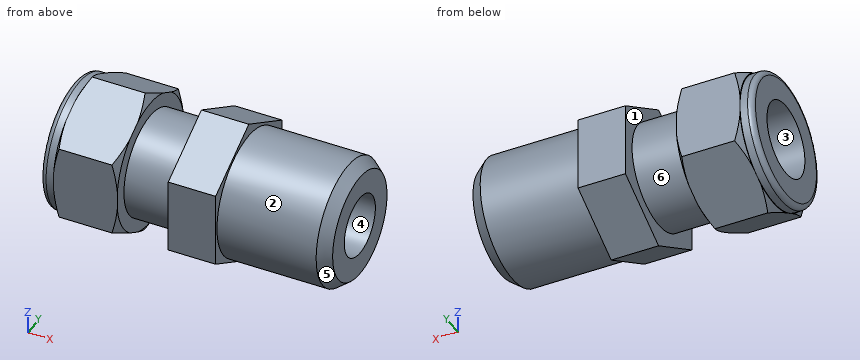
from build123d import *

# Parameters (mm, degrees)
HEX1_DEPTH         = 5.461
BODYFILLET_R       = 0.889
HEX2_DEPTH         = 8.128
DSCH_R             = 6.35
CUT_EXTRUDED_DEPTH = 22.86
SKETCH_E_R         = 5.207
CUT_EXTRUDEE_DEPTH = 26.162


with BuildPart() as part:
    # BodySch → Body (revolve)
    with BuildSketch(Plane.XY, mode=Mode.PRIVATE) as body_sk:
        Polygon((-49.022, 0), (-49.022, 11.1125), (-41.3766, 11.1125), (-41.3766, 8.89), (-27.178, 8.89), (-27.178, 10.668), (-2.033448841, 10.668), (0, 9.107679825), (0, 0), align=None)
    revolve(body_sk.sketch.rotate(Axis((-103.68469285, 0, 0), (1, 0, 0)), 90), axis=Axis((-103.68469285, 0, 0), (1, 0, 0)))

    # Hex1Sch_G → Hex1 (add, symmetric)
    with BuildSketch(Plane(origin=(-41.3766, 0, 0), x_dir=(0, 0, -1), z_dir=(1, 0, 0))):
        Polygon((12.831609733, 0), (6.415804866, 11.1125), (-6.415804866, 11.1125), (-12.831609733, 0), (-6.415804866, -11.1125), (6.415804866, -11.1125), align=None)
    extrude(amount=HEX1_DEPTH, both=True)

    # BodyFillet
    bodyfillet_edges = [part.edges().sort_by_distance(p)[0] for p in [
        (-49.022, 0, -11.1125),
    ]]
    fillet(bodyfillet_edges, radius=BODYFILLET_R)

    # HexfilletSch → Hexfillet (revolve, cut)
    with BuildSketch(Plane(origin=(0, 0, 0), x_dir=(1, 0, 0), z_dir=(0, 1, 0)), mode=Mode.PRIVATE) as hexfillet_sk:
        Polygon((-46.8376, 11.227658516), (-45.911558333, 12.831609733), (-46.8376, 12.831609733), align=None)
        Polygon((-35.9156, 11.227658516), (-36.841641667, 12.831609733), (-35.9156, 12.831609733), align=None)
    revolve(hexfillet_sk.sketch.rotate(Axis((-41.994761709, 0, 0), (1, 0, 0)), 150), axis=Axis((-41.994761709, 0, 0), (1, 0, 0)), mode=Mode.SUBTRACT)

    # Hex2Sch_F → Hex2 (add)
    with BuildSketch(Plane.ZY.offset(27.178)):
        Polygon((12.831609733, 0), (6.415804866, 11.1125), (-6.415804866, 11.1125), (-12.831609733, 0), (-6.415804866, -11.1125), (6.415804866, -11.1125), align=None)
    extrude(amount=-HEX2_DEPTH)

    # DSch → Cut-ExtrudeD (cut)
    with BuildSketch(Plane(origin=(-49.022, 0, 0), x_dir=(0, 0, -1), z_dir=(1, 0, 0))):
        Circle(DSCH_R)
    extrude(amount=CUT_EXTRUDED_DEPTH, mode=Mode.SUBTRACT)

    # Sketch E → Cut-ExtrudeE (cut)
    with BuildSketch(Plane(origin=(0, 0, 0), x_dir=(0, 0, -1), z_dir=(1, 0, 0))):
        Circle(SKETCH_E_R)
    extrude(amount=-CUT_EXTRUDEE_DEPTH, mode=Mode.SUBTRACT)


solid = part.part
Check sheet for the modelled part. Datum: model origin and axes. Units: mm. Face numbers are marked on the shaded views. A direction names the side the tool comes from. Round coordinates to 2 decimals unless told otherwise and drop trailing zeros. Write each loop counter-clockwise with the first axis right and the second up, starting at its lowest first coordinate (ties: lowest second). Pieces come first, ordered by that corner, then holes. Notation, with made-up numbers: (14.25, 83) - (21.25, 83) arc R14 ccw to (21.25, 106) - close; hole circle Ø10 at (23, 67). An arc over 180 degrees is marked (long way). Return JSON: item names as keys, results as strings.
Q1. Depth check by flat-ended pin: P1, Ø12, axis at x = -36, z = -4.5, coming from the -Y side; P2, Ø11.5, axis at y = 0, z = 0, coming from the -X side; P3, Ø12, axis at x = -42.5, y = 8.5, coming from the -Z side; P4, Ø1, axis at x = -27.5, y = 5, coming from the +Z side. Enter the tip coordinate at first touch or a pass-through.
Returned:
{"P1": "stops at y = -11.11", "P2": "stops at x = -26.16", "P3": "stops at z = -11.39", "P4": "stops at z = 10.17"}
Q2. Cross-section at B-B (x = -9). Record the boundary of the cut face in (y, z), then the cut area to 3 significant figures.
Returned:
{"outline": "circle Ø21.34 at (0, 0); hole circle Ø10.41 at (0, 0)", "area": "272 mm²"}
Q3. Scan lines: L1, parallel to Y at x = -10.5, z = -0.25; L2, parallel to Y at x = -20, z = 0; L3, parallel to X at y = -2.25, z = -4.75. Record each from-to range of solid material in increasing order. Write a range as from..to.
Returned:
{"L1": "y = -10.67..-5.2, 5.2..10.67", "L2": "y = -11.11..-5.21, 5.21..11.11", "L3": "x = -26.16..0"}
Q4. Access from +Z, -Z, +X, -X, +Y, -Y to the whole of each face (thin tool, end or side, straight path). Record for the marked faces 1, 2 and 3.
Returned:
{"face 1": "none", "face 2": "+X", "face 3": "-X"}
Q5. Draft check along X on the marked faces 4, 5 and 6. Enter one of: released by +X, released by -X, zero draft, split by the parting line, or undercut.
Returned:
{"face 4": "zero draft", "face 5": "released by +X", "face 6": "undercut"}
Q6. Cross-section at A-A (x = -42). Record the boundary of the cut face in (y, z).
Returned:
{"outline": "(-11.11, -6.42) - (0, -12.83) - (11.11, -6.42) - (11.11, 6.42) - (0, 12.83) - (-11.11, 6.42) - close; hole circle Ø12.7 at (0, 0)"}
